Answer from the drawing. Dimensions are ordinates in mm from the lowest x, y and z of the part. A direction names the side the tool comes from. Give positions to 0.01 mm unless a question says otherwise; leave off trailing zeros. Loops run counter-clockwise (first coordinate to the right, second up) from the corner with the lowest first, then second, coordinate; pieces in that order, holes last.
(1) Straight lines are drawn through the part: probe 1 along X at (y, z) = (35.5, 10.2); probe 2 along Z at (x, y) = (17.8, 13.75); probe 3 along Z at (x, y) = (31.5, 9). For each, find the intervals that lie inside material, in ascending order.
(2) Find section B-B, the plane z = 12. Write down the section's boundary in (x, y).
(3) Each of these flat-tipped pins is pushed along its axis until it touches: P1, Ø3, axis at x = 15.5, y = 10, coming from the +Z side; P2, Ø5, axis at x = 4, y = 22, coming from the +Z side; P3, Ø0.5, axis at y = 33.5, z = 9.5, coming from the -X side. Where does it stop, or does it pass through?
(4) Find section C-C, the plane y = 7.5. Write down the section's boundary in (x, z).
(5) Find section A-A, the plane x = 17.8. Write down the section's boundary in (y, z), then the cut area to 3 significant figures.
(6) Find section D-D, the plane x = 3. Write down the section's boundary in (y, z), then the cut area to 3 significant figures.
(7) Which of the six approach directions +Z, -Z, +X, -X, +Y, -Y give full straight-line access (tool end or side, diameter ignored) to the marked faces 1, 2 and 3?
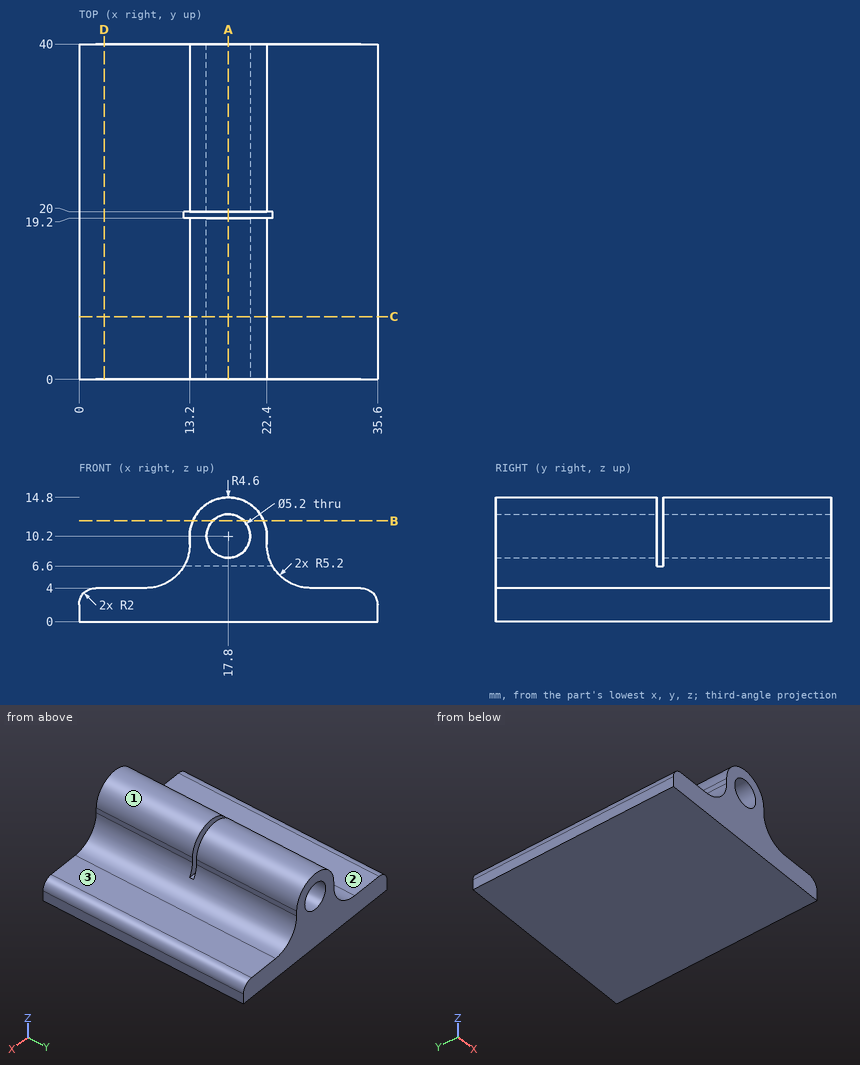
Entries:
1. probe 1: x = 13.2 to 15.2, 20.4 to 22.4
1. probe 2: z = 0 to 7.6, 12.8 to 14.8
1. probe 3: z = 0 to 4
2. outline: (13.57, 0) - (15.92, 0) - (15.92, 19.2) - (13.57, 19.2) - close; (13.57, 20) - (15.92, 20) - (15.92, 40) - (13.57, 40) - close; (19.68, 0) - (22.03, 0) - (22.03, 19.2) - (19.68, 19.2) - close; (19.68, 20) - (22.03, 20) - (22.03, 40) - (19.68, 40) - close
3. P1: stops at z = 14.73
3. P2: stops at z = 4
3. P3: stops at x = 13.2
4. outline: (0, 0) - (35.6, 0) - (35.6, 2) arc R2 ccw to (33.6, 4) - (27.6, 4) arc R5.2 cw to (22.4, 9.2) - (22.4, 10.2) arc R4.6 ccw to (13.2, 10.2) - (13.2, 9.2) arc R5.2 cw to (8, 4) - (2, 4) arc R2 ccw to (0, 2) - close; hole circle Ø5.2 at (17.8, 10.2)
5. outline: (0, 0) - (40, 0) - (40, 7.6) - (20, 7.6) - (20, 6.6) - (19.2, 6.6) - (19.2, 7.6) - (0, 7.6) - close; (0, 12.8) - (19.2, 12.8) - (19.2, 14.8) - (0, 14.8) - close; (20, 12.8) - (40, 12.8) - (40, 14.8) - (20, 14.8) - close
5. area: 382 mm2
6. outline: (0, 0) - (40, 0) - (40, 4) - (0, 4) - close
6. area: 160 mm2
7. face 1: +Z, +Y, -Y
7. face 2: +Z, -X, +Y, -Y
7. face 3: +Z, +X, +Y, -Y
